```python
from build123d import *

# Parameters (mm, degrees)
F0_R     = 20.32
F1_DEPTH = 19.812
F2_R     = 18.6937497488
F2_R_2   = 8.9962892538
F3_DEPTH = 2.54
F5_D     = 4.2
F5_DEPTH = 11.925
F5_TIP   = 1.2618073


with BuildPart() as f1:
    # F0 (on Front) → F1 (new body)
    with BuildSketch(Plane.XZ):
        Circle(F0_R)
    extrude(amount=F1_DEPTH)

    # F2 (on face) → F3 (cut)
    with BuildSketch(Plane.XZ.offset(19.812)):
        Circle(F2_R)
        Circle(F2_R_2, mode=Mode.SUBTRACT)
    extrude(amount=-F3_DEPTH, mode=Mode.SUBTRACT)

    # F5
    with Locations(Plane(origin=(0, 0, 0), x_dir=(-1, 0, 0), z_dir=(0, 1, 0))):
        with Locations((0, 0)):
            Hole(F5_D / 2, depth=F5_DEPTH)
            with Locations((0, 0, -(F5_DEPTH + F5_TIP / 2))):  # 118° drill point
                Cone(0, F5_D / 2, F5_TIP, mode=Mode.SUBTRACT)


solid = f1.part
```
Check sheet for the modelled part. Datum: model origin and axes. Units: mm. A direction names the side the tool comes from. Round coordinates to 2 decimals unless told otherwise and drop trailing zeros. Write each loop counter-clockwise with the first axis right and the second up, starting at its lowest first coordinate (ties: lowest second). Pieces come first, ordered by that corner, then holes. Notation, with made-up numbers: (-22.5, 68.25) -> (26.5, 68.25) arc R18 cw to (26.5, 90.25) -> close; hole circle Ø7 at (-31.75, 52). An arc over 180 degrees is marked (long way). Put each result on its own line as item: value.
(1) Sectioned sample at C-C (x = -14). Enter the section's corners in (y, z), plus the area to 3 significant figures.
Values found:
outline: (-19.81, -14.73) -> (0, -14.73) -> (0, 14.73) -> (-19.81, 14.73) -> (-19.81, 12.39) -> (-17.27, 12.39) -> (-17.27, -12.39) -> (-19.81, -12.39) -> close
area: 521 mm^2
(2) Sectioned sample at D-D (y = -15.25). Enter the section's corners in (x, z).
Values found:
outline: circle Ø40.64 at (0, 0)
(3) Tool access check on faces 4 (the face through (8.58, -18.56, 2.7)), 5 (the face through (18, -19.812, -6)). Record the directions out of +Z, -Z, +X, -X, +Y, -Y that give a thin tool (end or side, any length) a straight path to the whole face; none if there is none.
Values found:
face 4: -Y
face 5: +Z, -Z, +X, -X, -Y
(4) Go/stop test with flat-tipped pins: pin 1 Ø2 at (x, y) = (14, -2) entering from -Z; pin 2 Ø4 at (x, y) = (-3.5, -13.5) entering from -Z; pin 3 Ø1.5 at (y, z) = (-12, -12) entering from -X. Record where each tip stops, or that it passes through.
Values found:
pin 1: stops at z = -15.62
pin 2: stops at z = -20.26
pin 3: stops at x = -16.92
(5) Sectioned sample at B-B (y = -6.75). Enter the section's corners in (x, z), plus the area to 3 significant figures.
Values found:
outline: circle Ø40.64 at (0, 0); hole circle Ø4.2 at (0, 0)
area: 1,280 mm^2
(6) Material ranges on line 1 (Z direction, x = 0, y = -17.75); line 2 (Z direction, x = 0, y = -3); line 3 (Y direction, x = 0, z = 10), recorded low to high.
Values found:
line 1: z = -20.32 to -18.69, -9 to 9, 18.69 to 20.32
line 2: z = -20.32 to -2.1, 2.1 to 20.32
line 3: y = -17.27 to 0
(7) Mould release check, pull along X, two halves, no side actions. Record for faces 1 (the face through (2.003, -6.046, 0.631)), 2 (the face through (-2.645, -9.767, 20.147)), 3 (the face through (4, 0, 0)): released by +X, released by -X, zero draft, split by the parting line, or undercut.
Values found:
face 1: undercut
face 2: split by the parting line
face 3: zero draft
(8) Sectioned sample at A-A (z = 16). Enter the section's corners in (x, y).
Values found:
outline: (-12.53, -19.81) -> (-9.67, -19.81) -> (-9.67, -17.27) -> (9.67, -17.27) -> (9.67, -19.81) -> (12.53, -19.81) -> (12.53, 0) -> (-12.53, 0) -> close
